Print and shaded views of the part. All mm, measured from the part's lowest x, y and z. Round coordinates to 2 decimals unless told otherwise and drop trailing zeros. Write each loop counter-clockwise with the first axis right and the second up, starting at its lowest first coordinate (ties: lowest second). Pieces come first, ordered by that corner, then holes. Notation, with made-up numbers: M 16,70.25 L 34,70.25 A15 ccw 34,87.25 Z; hole C 27.25,46 d3. An arc over 180 degrees is marked long. Write item = value, one per line.
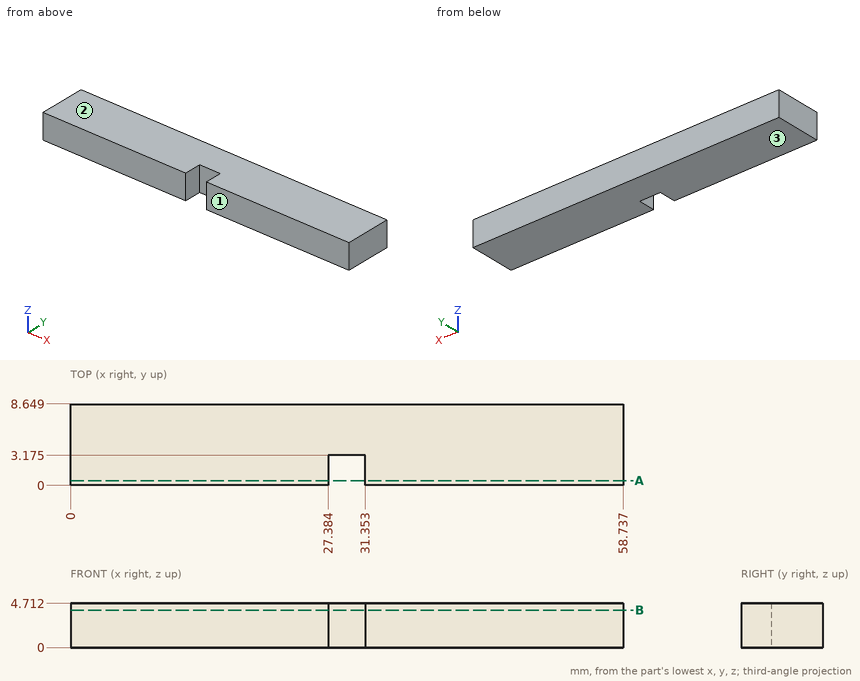
1. Band-saw the part on A-A (y = 0.5). List the corners of the cut face in (x, z) (1 decimal).
Responses:
outline = M 0,0 L 27.4,0 L 27.4,4.7 L 0,4.7 Z; M 31.4,0 L 58.7,0 L 58.7,4.7 L 31.4,4.7 Z
2. Probe probe 1 along X at (y, z) = (2, 1.6) (1 decimal); probe 2 along Y at (x, z) = (30, 4.25) (1 decimal). List the from-to ranges inside material, lowest first.
Responses:
probe_1 = 0 to 27.4, 31.4 to 58.7
probe_2 = 3.2 to 8.6
3. Mould opens along Z. For the marked faces 1, 2 and 3 say: pulls with the +Z half, pulls with the -Z half, needs draft (parallel to the pull), parting line crosses it, or undercut.
Responses:
face_1 = needs draft
face_2 = pulls with the +Z half
face_3 = pulls with the -Z half
4. Band-saw the part on B-B (z = 4). List the corners of the cut face in (x, y) (1 decimal).
Responses:
outline = M 0,0 L 27.4,0 L 27.4,3.2 L 31.4,3.2 L 31.4,0 L 58.7,0 L 58.7,8.6 L 0,8.6 Z
